from build123d import *

# Parameters (mm, degrees)
F0_W     = 30.48
F0_H     = 30.48
F0_W_2   = 26.67
F0_H_2   = 26.67
F1_DEPTH = 2.286
F2_DEPTH = 3.81
F10_R    = 6.35


with BuildPart() as f1:
    # F0 (on Top) → F1 (new body)
    with BuildSketch(Plane.XY):
        Rectangle(F0_W, F0_H)
        Rectangle(F0_W_2, F0_H_2, mode=Mode.SUBTRACT)
    extrude(amount=-F1_DEPTH)

    # F0 (on Top) → F2 (join)
    with BuildSketch(Plane.XY):
        Rectangle(F0_W, F0_H)
        Rectangle(F0_W_2, F0_H_2, mode=Mode.SUBTRACT)
    extrude(amount=F2_DEPTH)

    # F5 (on face) → F6 section 0
    with BuildSketch(Plane.XY.offset(3.81)):
        Polygon((-13.335, 13.335), (-15.24, 15.24), (-15.24, -15.24), (-13.335, -13.335), align=None)
    # F4 (on offset) → F6 section 1
    with BuildSketch(Plane.XY.offset(16.51)):
        Polygon((-6.35, -6.35), (-6.35, 6.35), (-8.255, 8.255), (-8.255, -8.255), align=None)
    loft()

    # F5 (on face) → F7 section 0
    with BuildSketch(Plane.XY.offset(3.81)):
        Polygon((-15.24, -15.24), (15.24, -15.24), (13.335, -13.335), (-13.335, -13.335), align=None)
    # F4 (on offset) → F7 section 1
    with BuildSketch(Plane.XY.offset(16.51)):
        Polygon((8.255, -8.255), (6.35, -6.35), (-6.35, -6.35), (-8.255, -8.255), align=None)
    loft()

    # F5 (on face) → F8 section 0
    with BuildSketch(Plane.XY.offset(3.81)):
        Polygon((15.24, -15.24), (15.24, 15.24), (13.335, 13.335), (13.335, -13.335), align=None)
    # F4 (on offset) → F8 section 1
    with BuildSketch(Plane.XY.offset(16.51)):
        Polygon((8.255, 8.255), (6.35, 6.35), (6.35, -6.35), (8.255, -8.255), align=None)
    loft()

    # F5 (on face) → F9 section 0
    with BuildSketch(Plane.XY.offset(3.81)):
        Polygon((13.335, 13.335), (15.24, 15.24), (-15.24, 15.24), (-13.335, 13.335), align=None)
    # F4 (on offset) → F9 section 1
    with BuildSketch(Plane.XY.offset(16.51)):
        Polygon((-6.35, 6.35), (6.35, 6.35), (8.255, 8.255), (-8.255, 8.255), align=None)
    loft()

    # F10
    f10_edges = [f1.edges().sort_by_distance(p)[0] for p in [
        (-11.7475, -11.7475, 10.16),
        (11.7475, -11.7475, 10.16),
        (11.7475, 11.7475, 10.16),
        (-11.7475, 11.7475, 10.16),
    ]]
    fillet(f10_edges, radius=F10_R)


solid = f1.part
Part model, mm, in its own coordinate system. A direction names the side the tool comes from. Give positions to 0.01 mm unless a question says otherwise; leave off trailing zeros.
1) Two-plate mould, pull along X, no slides. Class faces 3 (the face through (-15.24, 0, 1)), 4 (the face through (0, -15.24, 1)), 5 (the face through (-13.335, 0, 1)): released by +X, released by -X, zero draft, split by the parting line, or undercut.
Resolved:
face 3: released by -X
face 4: zero draft
face 5: undercut
2) Pin check, flat tips, straight feed: pin 1 (4 mm diameter, centred on x = 12, y = 11.5, fed in from +Z); pin 2 (4 mm diameter, centred on y = 7, z = 9, fed in from +X); pin 3 (6 mm diameter, centred on x = 10.5, y = -7.5, fed in from +Z). Stop position of each tip, or through.
Resolved:
pin 1: stops at z = 9.88
pin 2: stops at x = 13.49
pin 3: stops at z = 15.81
3) Which spindle directions (+Z, -Z, +X, -X, +Y, -Y) get a long thin tool onto all of the face, cutting with end or side? Do faces 1 (the face through (0, 13.335, 1)), 2 (the face through (0, 15.24, 1)). Say none if no direction does.
Resolved:
face 1: -Z
face 2: +Z, -Z, +X, -X, +Y
4) Probe L1, parallel to Y at x = -5, z = -0.75 (3 decimals); L2, parallel to Y at x = -7, z = 11.75. List the from-to ranges inside material, lowest first.
Resolved:
L1: y = -15.24 to -13.335, 13.335 to 15.24
L2: y = -10.65 to -8.97, 8.97 to 10.65
